Design review of the part shown in the three views and the two pictorial views. Dimensions are in mm from the part's minimum x, y and z. A direction names the side the tool comes from. Give positions to 0.01 mm unless a question says otherwise; leave off trailing zeros. Order: outer loops, then holes, each group sorted by start corner. A loop starts at its lowest first (then second) coordinate and runs counter-clockwise, first axis right, second up.
Item 1: Machinability: for the marked faces 1, 2 and 3, which of the approach directions +Z, -Z, +X, -X, +Y, -Y give a long, thin tool a straight path to every point of the face, cutting with its end or side? Answer none if there is none.
Item 2: Consider section C-C (y = 18). Give the boundary of the cut face in (x, z), plus the area to 3 significant figures.
Item 3: The part is to be moulded in two halves that separate along Y. For the marked faces 4, 5 and 6, say which applies: released by +Y, released by -Y, zero draft, split by the parting line, or undercut.
Item 4: For P1, Ø9, axis at x = 25, y = 30, coming from the +Z side; P2, Ø6, axis at x = 28, y = 42, coming from the +Z side; P3, Ø10, axis at x = 40, z = 42.5, coming from the -Y side; P4, Ø8, axis at x = 45, y = 34.5, coming from the +Z side, all flat-tipped, find the tip position at first contact; note any pin that passes through.
Item 5: Consider section D-D (x = 44). Give the boundary of the cut face in (y, z), plus the area to 3 significant figures.
Item 6: Consider section B-B (x = 25). Give the boundary of the cut face in (y, z), plus the area to 4 significant figures.
Item 7: For probe 1 along Z at (x, y) = (25, 63.25); probe 2 along Y at (x, z) = (24, 21); probe 3 along Y at (x, z) = (4.5, 35), list the stretches that pass through material, from the lowest coordinate up.
Item 8: Consider section A-A (y = 30). Give the boundary of the cut face in (x, z).
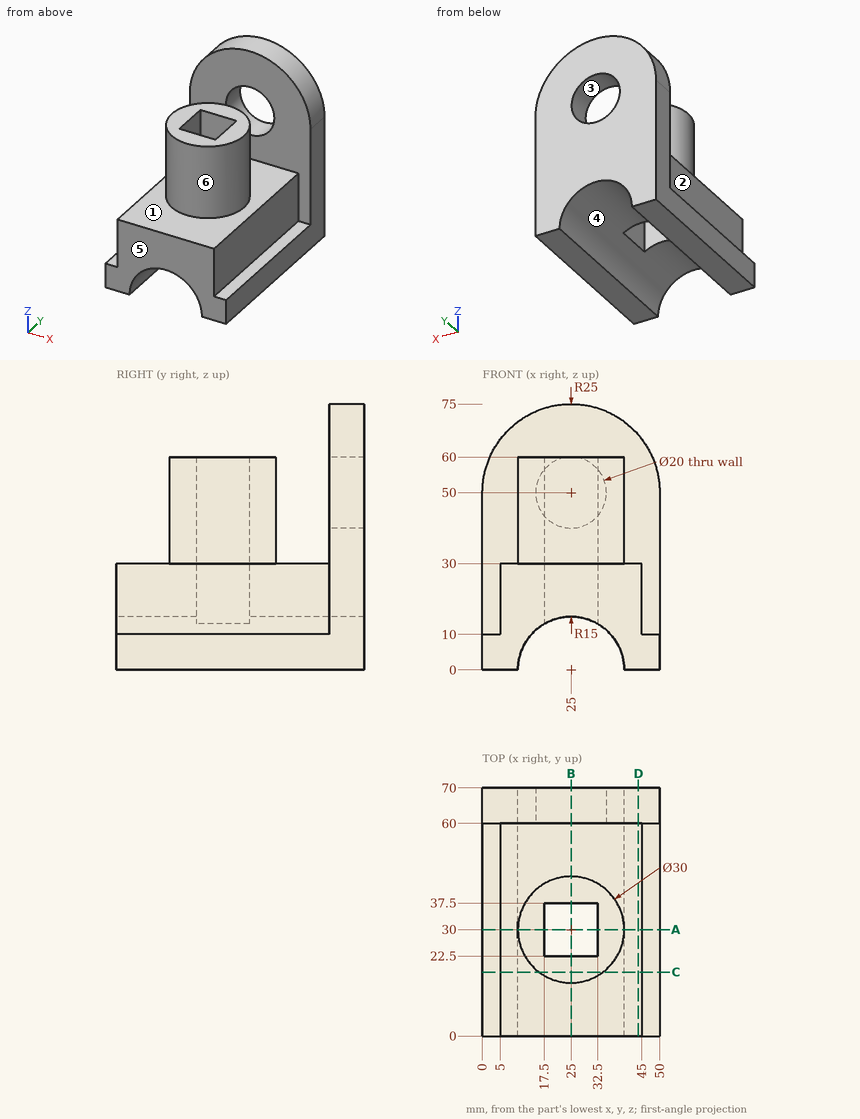
Resolved:
1. face 1: +Z
1. face 2: +Z, -X, -Y
1. face 3: +Y
2. outline: (0, 0) - (10, 0) arc R15 cw to (40, 0) - (50, 0) - (50, 10) - (45, 10) - (45, 30) - (34, 30) - (34, 60) - (16, 60) - (16, 30) - (5, 30) - (5, 10) - (0, 10) - close
2. area: 1,490 mm2
3. face 4: zero draft
3. face 5: released by -Y
3. face 6: undercut
4. P1: passes through
4. P2: stops at z = 60
4. P3: stops at y = 18.82
4. P4: stops at z = 30
5. outline: (0, 0) - (70, 0) - (70, 66.25) - (60, 66.25) - (60, 30) - (0, 30) - close
5. area: 2,460 mm2
6. outline: (0, 15) - (22.5, 15) - (22.5, 60) - (15, 60) - (15, 30) - (0, 30) - close; (37.5, 15) - (70, 15) - (70, 40) - (60, 40) - (60, 30) - (45, 30) - (45, 60) - (37.5, 60) - close; (60, 60) - (70, 60) - (70, 75) - (60, 75) - close
6. area: 1,525 mm2
7. probe 1: z = 15 to 40, 60 to 75
7. probe 2: y = 0 to 22.5, 37.5 to 70
7. probe 3: y = 60 to 70
8. outline: (0, 0) - (10, 0) arc R15 cw to (17.5, 12.99) - (17.5, 60) - (10, 60) - (10, 30) - (5, 30) - (5, 10) - (0, 10) - close; (32.5, 12.99) arc R15 cw to (40, 0) - (50, 0) - (50, 10) - (45, 10) - (45, 30) - (40, 30) - (40, 60) - (32.5, 60) - close
